Build history of the part. All positions in model axes, mm. A direction names the side the tool comes from. Round coordinates to 2 decimals unless told otherwise and drop trailing zeros. Write each loop counter-clockwise with the first axis right and the second up, starting at its lowest first coordinate (ties: lowest second). Pieces come first, ordered by that corner, then holes. Notation, with made-up numbers: M -31,59 L 22,59 A29 cw 22,86 Z; hole C 72,-4 d9. An arc over 180 degrees is marked long. Write item = value, one per line.
Autodesk Inventor part; units mm, degrees
ref_plane "YZ Plane" through (0, 0, 0) normal (1, 0, 0) x (0, 1, 0)
ref_plane "XZ Plane" through (0, 0, 0) normal (0, 1, 0) x (-1, 0, 0)
ref_plane "XY Plane" through (0, 0, 0) normal (0, 0, 1) x (1, 0, 0)
sketch "Sketch1" plane through (0, 0, 0) normal (0, 0, 1) x (1, 0, 0)
  line L0 (280, 0) -> (280, -1200)
  arc A0 (120, -1200) -> (280, -1200) centre (200, -1200) ccw
  line L1 (120, -1200) -> (120, 0)
  line L2 (-120, 0) -> (-120, -1200)
  arc A1 (-280, -1200) -> (-120, -1200) centre (-200, -1200) ccw
  line L3 (-280, -1200) -> (-280, 0)
  line L4 (280, 0) -> (-280, 0)
  line L5 (0, 0) -> (0, -1425.5319) construction
  dimension "d0" = 160
  dimension "d1" = 560
  dimension "d2" = 1200
extrude "Extrusion1" add sketch "Sketch1" along normal blind 100
sketch "Sketch2" plane through (0, 0, 100) normal (0, 0, 1) x (1, 0, 0)
  arc A0 (-280, -1200) -> (-120, -1200) centre (-200, -1200) ccw
  line L0 (-120, -1200) -> (-120, 0)
  line L1 (-120, 0) -> (-280, 0)
  line L2 (-280, 0) -> (-280, -1200)
  line L3 (280, 0) -> (120, 0)
  line L4 (120, 0) -> (120, -1200)
  arc A1 (120, -1200) -> (280, -1200) centre (200, -1200) ccw
  line L5 (280, -1200) -> (280, 0)
  line L6 (-280, -1060) -> (-200, -1060)
  line L7 (-200, -1060) -> (-200, -500)
  line L8 (-200, -500) -> (-280, -500)
  line L9 (-280, -500) -> (-280, -1060)
  line L10 (200, -1060) -> (280, -1060)
  line L11 (280, -1060) -> (280, -500)
  line L12 (280, -500) -> (200, -500)
  line L13 (200, -500) -> (200, -1060)
  line L14 (-200, -500) -> (200, -500)
  line L15 (200, -500) -> (200, -580)
  line L16 (200, -580) -> (-200, -580)
  line L17 (-200, -580) -> (-200, -500)
  line L18 (-280, 0) -> (-280, -1200)
  line L19 (280, -1200) -> (280, 0)
  point P0 (0, 0)
  point P1 (-200, -580)
  dimension "d5" = 80
  dimension "d6" = 560
  dimension "d7" = 560
  dimension "d8" = 400
  dimension "d9" = 500
extrude "Extrusion2" add sketch "Sketch2" along normal blind 40 contours L2 L8 L7 L6 | L16 L7 L14 L0 | L0 L14 L4 L16 | L4 L14 L13 L16 | L13 L12 L5 L10
sketch "Sketch3" plane through (0, 0, 140) normal (0, 0, 1) x (1, 0, 0)
  line L0 (-280, -500) -> (-280, -1060)
  line L1 (-280, -1060) -> (-200, -1060)
  line L2 (-200, -1060) -> (-200, -580)
  line L3 (-200, -580) -> (200, -580)
  line L4 (200, -580) -> (200, -1060)
  line L5 (200, -1060) -> (280, -1060)
  line L6 (280, -1060) -> (280, -500)
  line L7 (280, -500) -> (-280, -500)
  line L8 (-280, -1060) -> (-240, -1060)
  line L9 (-240, -1060) -> (-240, -1020)
  line L10 (-240, -1020) -> (-280, -1020)
  line L11 (-280, -1020) -> (-280, -1060)
  line L12 (-280, -500) -> (-240, -500)
  line L13 (-240, -500) -> (-240, -540)
  line L14 (-240, -540) -> (-280, -540)
  line L15 (-280, -540) -> (-280, -500)
  line L16 (280, -500) -> (240, -500)
  line L17 (240, -500) -> (240, -540)
  line L18 (240, -540) -> (280, -540)
  line L19 (280, -540) -> (280, -500)
  line L20 (280, -1060) -> (240, -1060)
  line L21 (240, -1060) -> (240, -1020)
  line L22 (240, -1020) -> (280, -1020)
  line L23 (280, -1020) -> (280, -1060)
  point P0 (0, 0)
  dimension "d12" = 40
extrude "Extrusion3" add sketch "Sketch3" along normal blind 60 contours L7 L13 L14 L0 | L10 L9 L1 L0 | L7 L6 L18 L17 | L6 L5 L21 L22
equation "\"d7\" = d6"
properties part number "pallet jack dummy_1200"
1. Band-saw the part on D-D (x = 144.5). List the corners of the cut face in (y, z).
Responses:
outline = M -1257.62,0 L 0,0 L 0,100 L -500,100 L -500,140 L -580,140 L -580,100 L -1257.62,100 Z
2. Flat gauge pins, fed straight in: pin 1 (2 mm diameter, centred on x = 180, z = 90.5, fed in from -Y); pin 2 (20 mm diameter, centred on x = -256.5, z = 166, fed in from +Y). Where does each tip first touch, or does it go through?
Responses:
pin_1 = -1277.71
pin_2 = -500
3. Band-saw the part on A-A (y = -978). List the corners of the cut face in (x, z), plus the area to 3 significant figures.
Responses:
outline = M -280,0 L -120,0 L -120,100 L -200,100 L -200,140 L -280,140 Z; M 120,0 L 280,0 L 280,140 L 200,140 L 200,100 L 120,100 Z
area = 38,400 mm²
4. Probe probe 1 along X at (y, z) = (-644, 55); probe 2 along X at (y, z) = (-769.5, 127); probe 3 along Z at (x, y) = (179.5, -318.5). List the from-to ranges inside material, lowest first.
Responses:
probe_1 = -280 to -120, 120 to 280
probe_2 = -280 to -200, 200 to 280
probe_3 = 0 to 100
5. Mould opens along X. For faces 1 (the face through (199, -631, 0)), 2 (the face through (280, -608, 54)), 3 (the face through (201.76, -1279.98, 49.3)), 4 (the face through (-22, -571, 140)) say: pulls with the +X half, pulls with the -X half, needs draft (parallel to the pull), parting line crosses it, or undercut.
Responses:
face_1 = needs draft
face_2 = pulls with the +X half
face_3 = undercut
face_4 = undercut
6. Band-saw the part on B-B (z = 36.5). List the corners of the cut face in (x, y).
Responses:
outline = M -280,-1200 A80 ccw -120,-1200 L -120,0 L -280,0 Z; M 120,-1200 A80 ccw 280,-1200 L 280,0 L 120,0 Z
7. Band-saw the part on C-C (y = -419.5). List the corners of the cut face in (x, z).
Responses:
outline = M -280,0 L -120,0 L -120,100 L -280,100 Z; M 120,0 L 280,0 L 280,100 L 120,100 Z
8. Tool access for faces 5 (the face through (4, -500, 127)), 6 (the face through (-249, -1060, 138)), 7 (the face through (-240, -1040, 170)), 8 (the face through (-2, -539, 100)): list every direction of +Z, -Z, +X, -X, +Y, -Y with a clear straight run to the whole face (end or side of a thin tool).
Responses:
face_5 = +Z, +X, -X, +Y
face_6 = +Z, +X, -X, -Y
face_7 = +Z, +Y, -Y
face_8 = -Z, +Y, -Y
